Input: dimensioned drawing with shaded views. Units: mm. Origin: part minimum x, y, z. A direction names the side the tool comes from. Round coordinates to 2 decimals unless told otherwise and drop trailing zeros. Order: outer loops, then holes, each group sorted by start corner. A loop starts at its lowest first (then second) coordinate and runs counter-clockwise, first axis right, second up. Notation, with made-up numbers: M 15.25,-27 L 24.25,-27 A15 ccw 24.25,-9 Z; hole C 23.25,7.5 d2. An arc over 180 degrees is marked long. Use one line per item in the form item = value. Start each with the question number.
Q1. Section B-B (y = 4.2). Return the cut outline in (x, z) (1 decimal).
Q2. Section C-C (z = 2.15). Return the cut outline in (x, y).
Q3. Contact query for flat-ended pins moving along their axis: pin 1 (0.6 mm diameter, centred on x = 4, y = 3.5, fed in from -Z); pin 2 (1.6 mm diameter, centred on x = 3, y = 3.5, fed in from +Z); pin 3 (0.6 mm diameter, centred on x = 3, z = 1.5, fed in from -Y). Output: stop coordinate, or through.
Q4. Material intervals for probe 1 along Y at (x, z) = (4, 1.35); probe 2 along Z at (x, y) = (2, 3.1); probe 3 along Z at (x, y) = (7.75, 1.75) (1 decimal), sorted ascending.
Q5. Reachability of the marked faces 1, 2 and 3 from +Z, -Z, +X, -X, +Y, -Y: full face, straight path, thin tool, end or side. Return the list, or none.
Q6. Section D-D (x = 2). Return the cut outline in (y, z).
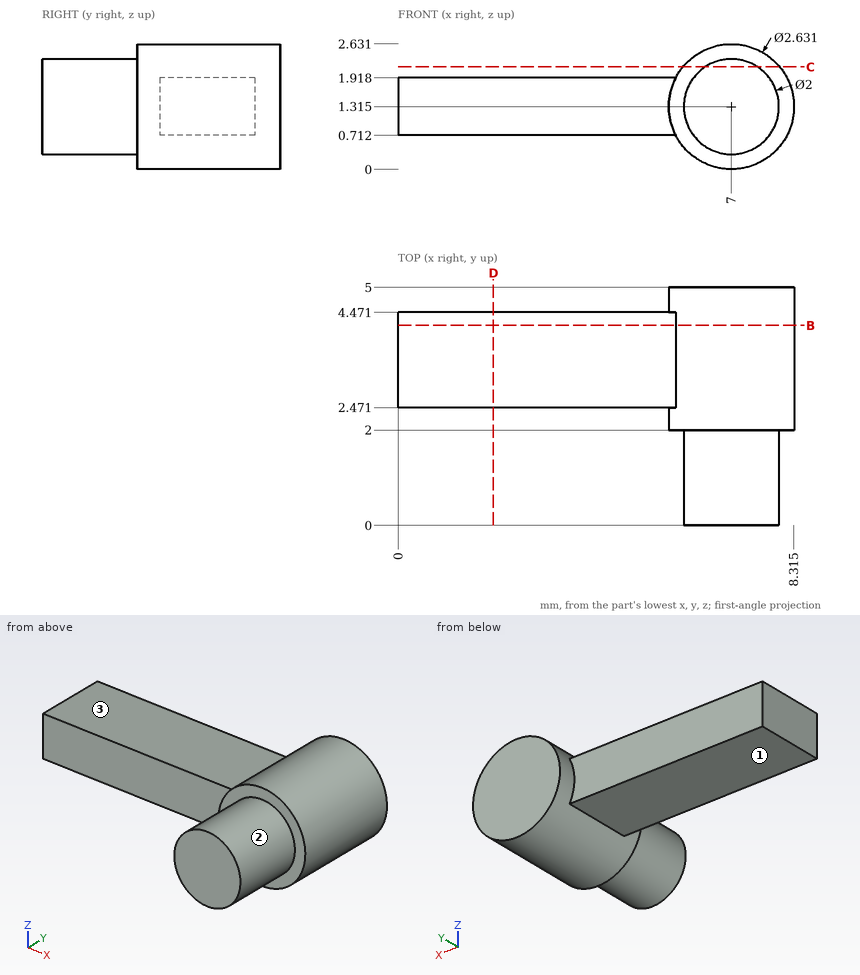
Results list:
q1.outline = M 0,0.7 L 5.8,0.7 A1.3 ccw long 5.8,1.9 L 0,1.9 Z
q2.outline = M 5.98,2 L 6.45,2 L 6.45,0 L 7.55,0 L 7.55,2 L 8.02,2 L 8.02,5 L 5.98,5 Z
q3.pin_1 = 0.71
q3.pin_2 = 1.92
q3.pin_3 = 2.47
q4.probe_1 = 2.47 to 4.47
q4.probe_2 = 0.71 to 1.92
q4.probe_3 = 0.7 to 2
q5.face_1 = -Z, -X, +Y, -Y
q5.face_2 = -Y
q5.face_3 = +Z, -X, +Y, -Y
q6.outline = M 2.47,0.71 L 4.47,0.71 L 4.47,1.92 L 2.47,1.92 Z
